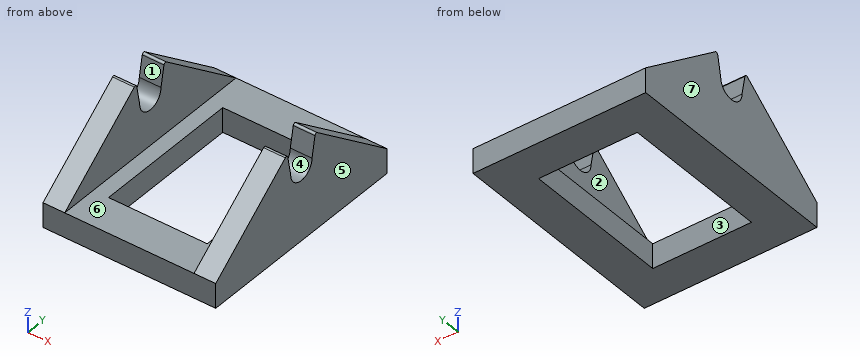
Autodesk Inventor part; units mm, degrees
ref_plane "YZ Plane" through (0, 0, 0) normal (1, 0, 0) x (0, 1, 0)
ref_plane "XZ Plane" through (0, 0, 0) normal (0, 1, 0) x (-1, 0, 0)
ref_plane "XY Plane" through (0, 0, 0) normal (0, 0, 1) x (1, 0, 0)
sketch "Sketch1" plane through (0, 0, 0) normal (0, 0, 1) x (1, 0, 0)
  line L0 (0, 0) -> (22.225, 0)
  line L1 (22.225, 0) -> (22.225, 28.575)
  line L2 (22.225, 28.575) -> (0, 28.575)
  line L3 (0, 28.575) -> (0, 0)
  line L4 (4.7625, 4.7625) -> (17.4625, 4.7625)
  line L5 (17.4625, 4.7625) -> (17.4625, 23.8125)
  line L6 (17.4625, 23.8125) -> (4.7625, 23.8125)
  line L7 (4.7625, 23.8125) -> (4.7625, 4.7625)
  point P0 (17.4625, 14.2875)
  point P1 (22.225, 14.2875)
  point P2 (11.1125, 23.8125)
  point P3 (11.1125, 28.575)
  dimension "d0" = 22.225
  dimension "d1" = 28.575
  dimension "d2" = 19.05
  dimension "d3" = 12.7
extrude "Extrusion1" add sketch "Sketch1" along normal blind 3.175
sketch "Sketch2" plane through (22.225, 0, 0) normal (1, 0, 0) x (0, 0, -1)
  line L0 (-3.175, 0) -> (-3.175, 28.575)
  arc A0 (-9.525, 12.5095) -> (-9.525, 16.0655) centre (-9.525, 14.2875) ccw
  arc A1 (-12.5246, 11.9383) -> (-12.5246, 16.6367) centre (-9.525, 14.2875) ccw
  line L1 (-3.175, 28.575) -> (-12.5246, 16.6367)
  line L2 (-3.175, 0) -> (-12.5246, 11.9383)
  line L3 (-12.5246, 11.9383) -> (-9.525, 12.5095)
  line L4 (-12.5246, 16.6367) -> (-9.525, 16.0655)
  point P0 (0, 0)
  point P1 (-3.175, 14.2875)
  dimension "d6" = 3.556
  dimension "d7" = 6.35
  dimension "d8" = 7.62
extrude "Extrusion2" add sketch "Sketch2" against normal blind 2.794
sketch "Sketch3" plane through (0, 0, 0) normal (-1, 0, 0) x (0, 0, 1)
  line L0 (3.175, 0) -> (3.175, 28.575)
  line L1 (3.175, 0) -> (12.5246, 11.9383)
  line L2 (12.5246, 11.9383) -> (9.525, 12.5095)
  arc A0 (9.525, 16.0655) -> (9.525, 12.5095) centre (9.525, 14.2875) ccw
  line L3 (9.525, 16.0655) -> (12.5246, 16.6367)
  line L4 (12.5246, 16.6367) -> (3.175, 28.575)
  point P0 (0, 0)
extrude "Extrusion3" add sketch "Sketch3" against normal blind 2.794
fillet "Fillet1" radius 0.254 4 edges at (1.397, 16.6367, 12.5246) (1.397, 11.9383, 12.5246) (20.828, 16.6367, 12.5246) (20.828, 11.9383, 12.5246)
properties part number "switchHolder"
Design review of the part built by this model. Coordinates are the model's own, in mm. Face numbers are marked on the shaded views. A direction names the side the tool comes from. Coordinates: 2 decimals unless noted, no trailing zeros. Order: outer loops, then holes, each group sorted by start corner. A loop starts at its lowest first (then second) coordinate and runs counter-clockwise, first axis right, second up. Notation, with made-up numbers: M -13.5,-29.5 L -9.5,-29.5 A21 cw -9.5,-14.5 Z; hole C 13,79.25 d4. An arc over 180 degrees is marked long. Answer as a JSON object with one key per item and string values. Group by question number.
1) Add section A-A, the plane x = 7. Write out the cut boundary in (y, z) (1 decimal), then the cut area to 3 significant figures.
2) Mouldability with a two-part tool opening along X and no side actions: class the marked faces 4, 5, 6 and 7 as pulls with the +X half, pulls with the -X half, needs draft (parallel to the pull), parting line crosses it, or undercut.
3) Tool access review of the marked faces 1, 2 and 3: name each direction out of +Z, -Z, +X, -X, +Y, -Y from which nothing blocks a thin tool from reaching the whole face with its end or side.
4) Add section C-C, the plane y = 18.75. Write out the cut boundary in (x, z) (1 decimal), then the cut area to 3 significant figures.
5) For pin 1 (3 mm diameter, centred on x = 2.5, z = 5.5, fed in from -Y); pin 2 (4 mm diameter, centred on x = 5, y = 11.5, fed in from +Z) (3 decimals); pin 3 (6 mm diameter, centred on x = 17, y = 21, fed in from +Z), all flat-tipped, find the tip position at first contact; note any pin that passes through.
6) Wall thickness on L1, parallel to X at y = 14.5, z = 6 (3 decimals); L2, parallel to X at y = 11, z = 1 (1 decimal); L3, parallel to Y at x = 5.75, z = 1.75 (1 decimal): over which ranges is each line inside the solid? List them lowest first.
7) Add section B-B, the plane z = 1. Write out the cut boundary in (x, y) (1 decimal).
8) Add section D-D, the plane z = 10. Write out the cut boundary in (x, y) (3 decimals).
Computed values:
{
 "1": {"outline": "M 0,0 L 4.8,0 L 4.8,3.2 L 0,3.2 Z; M 23.8,0 L 28.6,0 L 28.6,3.2 L 23.8,3.2 Z", "area": "30.2 mm^2"},
 "2": {"face 4": "needs draft", "face 5": "pulls with the +X half", "face 6": "undercut", "face 7": "pulls with the -X half"},
 "3": {"face 1": "+Z, +X, -X", "face 2": "+Z, +Y, -Y", "face 3": "+Z, -Z"},
 "4": {"outline": "M 0,0 L 4.8,0 L 4.8,3.2 L 2.8,3.2 L 2.8,10.9 L 0,10.9 Z; M 17.5,0 L 22.2,0 L 22.2,10.9 L 19.4,10.9 L 19.4,3.2 L 17.5,3.2 Z", "area": "73.2 mm^2"},
 "5": {"pin 1": "stops at y = 1.05", "pin 2": "stops at z = 3.175", "pin 3": "stops at z = 10.48"},
 "6": {"L1": "x = 0 to 2.794, 19.431 to 22.225", "L2": "x = 0 to 4.8, 17.5 to 22.2", "L3": "y = 0 to 4.8, 23.8 to 28.6"},
 "7": {"outline": "M 0,0 L 22.2,0 L 22.2,28.6 L 0,28.6 Z; hole M 4.8,4.8 L 17.5,4.8 L 17.5,23.8 L 4.8,23.8 Z"},
 "8": {"outline": "M 0,8.715 L 2.794,8.715 L 2.794,12.419 L 0,12.419 Z; M 0,16.156 L 2.794,16.156 L 2.794,19.86 L 0,19.86 Z; M 19.431,8.715 L 22.225,8.715 L 22.225,12.419 L 19.431,12.419 Z; M 19.431,16.156 L 22.225,16.156 L 22.225,19.86 L 19.431,19.86 Z"}
}
